Model file for the job. Use its own axes, mm. Face numbers are marked on the shaded views. A direction names the side the tool comes from. Round coordinates to 2 decimals unless told otherwise and drop trailing zeros. Order: outer loops, then holes, each group sorted by start corner. A loop starts at its lowest first (then second) coordinate and runs counter-clockwise, first axis right, second up. Notation, with made-up numbers: (57, -21) - (90, -21) arc R13 cw to (90, -9) - close; hole circle Ø6 at (60.5, -28.5). An arc over 180 degrees is marked (long way). Use one line per item in the form item = value.
Autodesk Inventor part; units mm, degrees
ref_plane "YZ Plane" through (0, 0, 0) normal (1, 0, 0) x (0, 1, 0)
ref_plane "XZ Plane" through (0, 0, 0) normal (0, 1, 0) x (-1, 0, 0)
ref_plane "XY Plane" through (0, 0, 0) normal (0, 0, 1) x (1, 0, 0)
sketch "Sketch1" plane through (0, 0, 0) normal (0, 1, 0) x (-1, 0, 0)
  circle A0 centre (0, 0) radius 7.5
  dimension "d0" = 15
extrude "Extrusion1" add sketch "Sketch1" along normal blind 1
sketch "Sketch2" plane through (0, 1, 0) normal (0, 1, 0) x (1, 0, 0)
  line L0 (-0.565, -6.85) -> (0.565, -6.85)
  line L1 (0.565, -6.85) -> (0.565, 6.85)
  line L2 (0.565, 6.85) -> (-0.565, 6.85)
  line L3 (-0.565, 6.85) -> (-0.565, -6.85)
  line L4 (-0.565, -6.85) -> (0.565, 6.85) construction
  line L5 (0.565, -6.85) -> (-0.565, 6.85) construction
  line L6 (6.85, -0.565) -> (-6.85, -0.565)
  line L7 (-6.85, -0.565) -> (-6.85, 0.565)
  line L8 (-6.85, 0.565) -> (6.85, 0.565)
  line L9 (6.85, 0.565) -> (6.85, -0.565)
  line L10 (6.85, -0.565) -> (-6.85, 0.565) construction
  line L11 (-6.85, -0.565) -> (6.85, 0.565) construction
  point P0 (0, 0)
  point P1 (0.565, 0.565)
  point P2 (-0.565, 0.565)
  point P3 (-0.565, -0.565)
  point P4 (0.565, -0.565)
  dimension "d3" = 13.7
  dimension "d4" = 13.7
  dimension "d5" = 1.13
  dimension "d6" = 1.13
extrude "Extrusion2" add sketch "Sketch2" along normal blind 83.3
sketch "Sketch3" plane through (0, 84.3, 0) normal (0, 1, 0) x (1, 0, 0)
  circle A0 centre (0, 0) radius 8.25
  dimension "d9" = 16.5
extrude "Extrusion3" add sketch "Sketch3" along normal blind 1.5
sketch "Sketch4" plane through (6.85, 1, -0.565) normal (1, 0, 0) x (0, 0, -1)
  line L0 (-1.13, 0) -> (-1.13, 83.3)
  line L1 (0, 0) -> (0, 83.3)
  line L2 (-1.13, 83.3) -> (0, 83.3)
  line L3 (0, 83.3) -> (0, 66.3)
  line L4 (0, 66.3) -> (-1.13, 66.3)
  line L5 (-1.13, 66.3) -> (-1.13, 83.3)
  point P0 (-0.565, -1)
  dimension "d12" = 17
extrude "Extrusion4" cut sketch "Sketch4" against normal blind 2
pattern_circular "Circular Pattern1" count 4 over 360 about axis through (0, 84.3, 0) along (0, 1, 0) of "Extrusion4"
fillet "Fillet1" radius 5 8 edges at (4.85, 67.3, 0) (0, 67.3, -4.85) (-4.85, 67.3, 0) (0, 67.3, 4.85) (-6.85, 67.3, 0) (0, 67.3, 6.85) (0, 67.3, -6.85) (6.85, 67.3, 0)
fillet "Fillet2" radius 2 4 edges at (0, 84.3, -4.85) (-4.85, 84.3, 0) (0, 84.3, 4.85) (4.85, 84.3, 0)
fillet "Fillet3" radius 0.5 2 edges at (-8.25, 84.3, 0) (-8.25, 85.8, 0)
sketch "Sketch6" plane through (0, 0, 0) normal (0, 0, 1) x (1, 0, 0)
  line L0 (-7.7, 0) -> (-7.7, -4.8)
  line L1 (-7.7, -4.8) -> (0, -7.8)
  line L2 (0, -7.8) -> (0, 0)
  line L3 (0, 0) -> (-7.7, 0)
  line L4 (0, -26.52) -> (0, 104.52)
  dimension "d22" = 4.8
  dimension "d23" = 7.7
  dimension "d24" = 3
revolve "Revolution1" add sketch "Sketch6" angle 360 about axis through (0, 0, 0) along (0, 1, 0)
properties part number "10 mL syringe plunger"
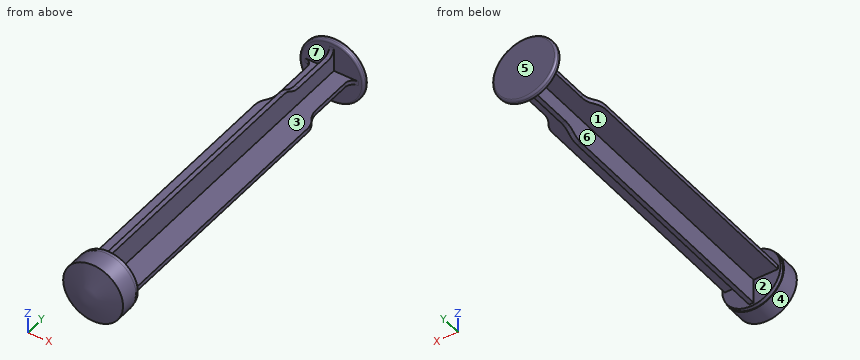
(1) Tool access for the marked faces 1, 2 and 3: list every direction of +Z, -Z, +X, -X, +Y, -Y with a clear straight run to the whole face (end or side of a thin tool).
Report:
face_1 = -Z, -X
face_2 = none
face_3 = +Z, +X
(2) Pin check, flat tips, straight feed: pin 1 (0.9 mm diameter, centred on y = 76, z = 0, fed in from +X); pin 2 (2 mm diameter, centred on x = -6, z = 5.5, fed in from -Y); pin 3 (1.2 mm diameter, centred on y = 34.5, z = 0, fed in from +X). Stop position of each tip, or through.
Report:
pin_1 = 4.85
pin_2 = -5.02
pin_3 = 6.85
(3) Slice it at B-B on y = 75.5. Give the cut face in (x, z) (3 decimals).
Report:
outline = (-4.85, -0.565) - (-0.565, -0.565) - (-0.565, -4.85) - (0.565, -4.85) - (0.565, -0.565) - (4.85, -0.565) - (4.85, 0.565) - (0.565, 0.565) - (0.565, 4.85) - (-0.565, 4.85) - (-0.565, 0.565) - (-4.85, 0.565) - close
(4) Pull direction Y, two halves, no side cores. Call the marked faces 4, 5, 6 and 7: released by +Y, released by -Y, zero draft, split by the parting line, or undercut.
Report:
face_4 = zero draft
face_5 = released by +Y
face_6 = undercut
face_7 = undercut
(5) Probe probe 1 along X at (y, z) = (62, 2) (3 decimals); probe 2 along Y at (x, z) = (5, 4). List the from-to ranges inside material, lowest first. Write a range as [from, to].
Report:
probe_1 = [-0.565, 0.565]
probe_2 = [-5.31, 1], [84.3, 85.8]
(6) Slice it at A-A on y = 49.5. Give the cut face in (x, z) (3 decimals).
Report:
outline = (-6.85, -0.565) - (-0.565, -0.565) - (-0.565, -6.85) - (0.565, -6.85) - (0.565, -0.565) - (6.85, -0.565) - (6.85, 0.565) - (0.565, 0.565) - (0.565, 6.85) - (-0.565, 6.85) - (-0.565, 0.565) - (-6.85, 0.565) - close
